Here's the drawing with two shaded views (mm, measured from the low corner). I have some questions. A direction names the side the tool comes from. Coordinates: 2 decimals unless noted, no trailing zeros. Order: outer loops, then holes, each group sorted by start corner. A loop starts at its lowest first (then second) coordinate and runs counter-clockwise, first axis right, second up. Notation, with made-up numbers: (-13.5, 71.25) - (6.5, 71.25) arc R26 cw to (6.5, 106.25) - close; hole circle Ø4 at (24, 45.25). An arc over 180 degrees is marked (long way). Answer as CSV lines item,"result". Start each with the question number.
1. Thinking about a two-plate mould opening in Z: for the marked faces 6, 7 and 8, which applies, released by +Z, released by -Z, zero draft, split by the parting line, or undercut?
2. I want a section at D-D, the plane z = 12.25. List the corners of the cut face in (x, y) for me, and give its area (3 significant figures).
3. I want a section at B-B, the plane y = 20.5. List the corners of the cut face in (x, z) for me.
4. I want a section at C-C, the plane x = 8.75. List the corners of the cut face in (y, z) for me, and give its area (3 significant figures).
5. I need wall thicknesses on probe 1 along X at (y, z) = (3.75, 5.75); probe 2 along X at (y, z) = (1.65, 7.5); probe 3 along X at (y, z) = (1, 7.5). Which ranges of each line are inside material? Lowest first, please.
6. For the marked faces 1, 2, 3, 4 and 5, which set-ups out of +Z, -Z, +X, -X, +Y, -Y let a thin tool reach every point of the face, with its end or its side?
7. I want a section at A-A, the plane z = 7.5. List the corners of the cut face in (x, y) for me, and give its area (3 significant figures).
8. For pin 1 (3 mm diameter, centred on y = 11, z = 2.5, fed in from -X); pin 2 (4.5 mm diameter, centred on y = 15, z = 9.5, fed in from +X); pin 3 (4 mm diameter, centred on x = 64, z = 4, fed in from +Y); pin 4 (1.8 mm diameter, centred on x = 65.25, z = 7.5, fed in from -Y), each with a flat end and sliding along its axis, tell me the tip position at first contact or that it passes through.
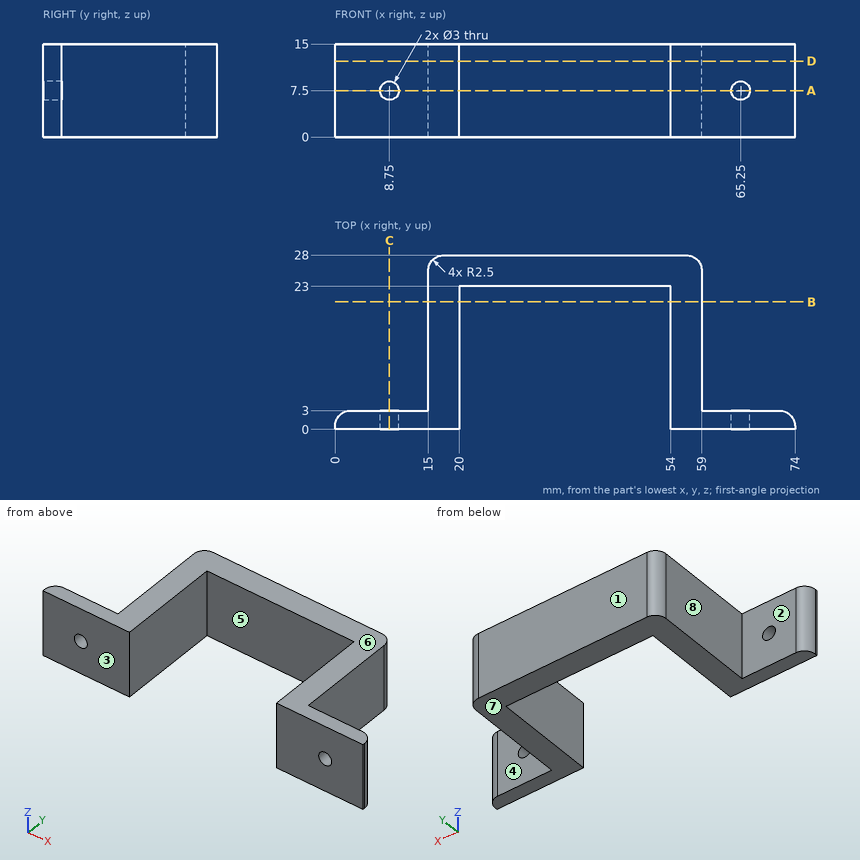
Solved:
1,face 6,"released by +Z"
1,face 7,"released by -Z"
1,face 8,"zero draft"
2,outline,"(0, 0) - (20, 0) - (20, 23) - (54, 23) - (54, 0) - (74, 0) - (74, 0.5) arc R2.5 ccw to (71.5, 3) - (59, 3) - (59, 25.5) arc R2.5 ccw to (56.5, 28) - (17.5, 28) arc R2.5 ccw to (15, 25.5) - (15, 3) - (2.5, 3) arc R2.5 ccw to (0, 0.5) - close"
2,area,"535 mm2"
3,outline,"(15, 0) - (20, 0) - (20, 15) - (15, 15) - close; (54, 0) - (59, 0) - (59, 15) - (54, 15) - close"
4,outline,"(0, 0) - (3, 0) - (3, 6) - (0, 6) - close; (0, 9) - (3, 9) - (3, 15) - (0, 15) - close"
4,area,"36.0 mm2"
5,probe 1,"x = 15 to 20, 54 to 59"
5,probe 2,"x = 0.28 to 7.25, 10.25 to 20, 54 to 63.75, 66.75 to 73.72"
5,probe 3,"x = 0.05 to 7.25, 10.25 to 20, 54 to 63.75, 66.75 to 73.95"
6,face 1,"+Z, -Z, +X, -X, +Y"
6,face 2,"+Z, -Z, -X, +Y"
6,face 3,"+Z, -Z, +X, -X, -Y"
6,face 4,"+Z, -Z, +X, +Y"
6,face 5,"+Z, -Z, -Y"
7,outline,"(0, 0) - (7.25, 0) - (7.25, 3) - (2.5, 3) arc R2.5 ccw to (0, 0.5) - close; (10.25, 0) - (20, 0) - (20, 23) - (54, 23) - (54, 0) - (63.75, 0) - (63.75, 3) - (59, 3) - (59, 25.5) arc R2.5 ccw to (56.5, 28) - (17.5, 28) arc R2.5 ccw to (15, 25.5) - (15, 3) - (10.25, 3) - close; (66.75, 0) - (74, 0) - (74, 0.5) arc R2.5 ccw to (71.5, 3) - (66.75, 3) - close"
7,area,"517 mm2"
8,pin 1,"stops at x = 15"
8,pin 2,"stops at x = 59"
8,pin 3,"stops at y = 3"
8,pin 4,"passes through"
